Can you work these out from the drawing? Everything is in mm from the part's minimum corner. Round coordinates to 2 decimals unless told otherwise and drop trailing zeros. Loops run counter-clockwise (first coordinate to the right, second up) from the corner with the lowest first, then second, coordinate; pieces in that order, holes last. Notation, with made-up numbers: (20, -1.5) - (26, -1.5) arc R24 cw to (26, 27.5) - close; hole circle Ø10 at (-14, 25.25). An arc over 180 degrees is marked (long way). Answer as a JSON object with one key per item and string values. Group by question number.
1) I want a section at C-C, the plane y = 144. Please give me the cut outline in (x, z), then the cut area to 3 significant figures.
2) If I drill on line 1 along X through (y, z) = (197.5, 8.5); line 2 along Y through (x, z) = (150.5, 7.5); line 3 along X through (y, z) = (317.5, 9), over which ranges is the centre line in solid material (lowest first)? Write a range as [from, to].
3) I want a section at D-D, the plane x = 47.5. Please give me the cut outline in (y, z), then the cut area to 3 significant figures.
4) I want a section at B-B, the plane z = 8. Please give me the cut outline in (x, y).
5) Will these pins go through, and if not, where does the flat tip stop? P1, Ø5, axis at y = 167.5, z = 14.5, coming from the -X side; P2, Ø1, axis at y = 133, z = 9, coming from the +X side; P3, Ø8, axis at y = 95.5, z = 5.5, coming from the -X side.
6) I want a section at A-A, the plane x = 100. Please give me the cut outline in (y, z).
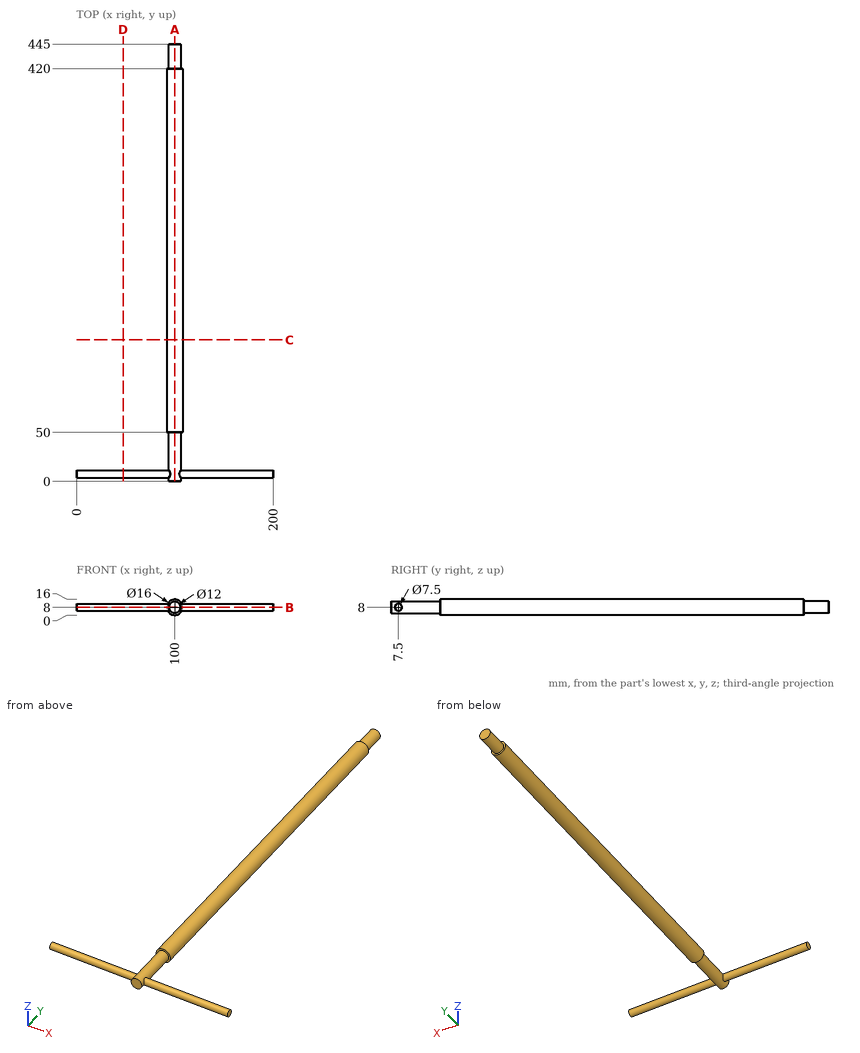
Outcome:
{
 "1": {"outline": "circle Ø16 at (100, 8)", "area": "201 mm^2"},
 "2": {"line 1": "[92.02, 107.98]", "line 2": "[3.78, 11.22]", "line 3": "[92.06, 107.94]"},
 "3": {"outline": "circle Ø7.5 at (7.5, 8)", "area": "44.2 mm^2"},
 "4": {"outline": "(0, 3.75) - (94, 3.75) - (94, 0) - (106, 0) - (106, 3.75) - (200, 3.75) - (200, 11.25) - (106, 11.25) - (106, 50) - (108, 50) - (108, 420) - (106, 420) - (106, 445) - (94, 445) - (94, 420) - (92, 420) - (92, 50) - (94, 50) - (94, 11.25) - (0, 11.25) - close"},
 "5": {"P1": "x = 93.07", "P2": "x = 107.98", "P3": "x = 92"},
 "6": {"outline": "(0, 2) - (50, 2) - (50, 0) - (420, 0) - (420, 2) - (445, 2) - (445, 14) - (420, 14) - (420, 16) - (50, 16) - (50, 14) - (0, 14) - close"}
}
